Work out the finished part from the listing and answer in its coordinate system (mm). Face numbers are marked on the shaded views. A direction names the side the tool comes from. Round coordinates to 2 decimals unless told otherwise and drop trailing zeros. Loops run counter-clockwise (first coordinate to the right, second up) from the corner with the lowest first, then second, coordinate; pieces in that order, holes last. Notation, with made-up numbers: (56.25, 19.25) -> (64.25, 19.25) arc R19 ccw to (64.25, 54.25) -> close; hole circle Ø4 at (-29, 4). An arc over 180 degrees is marked (long way). Use one line per item in the form item = value.
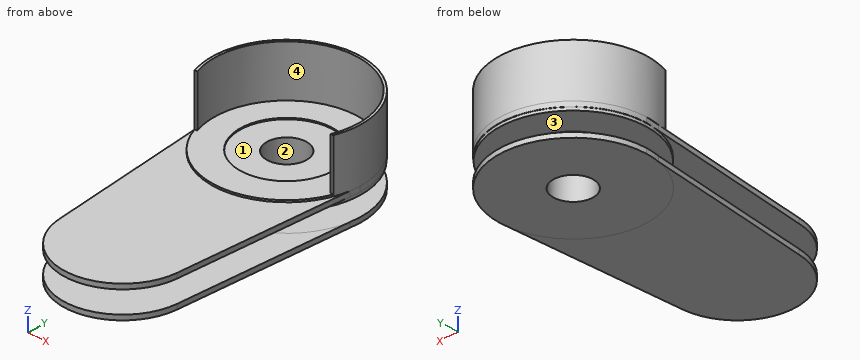
```python
from build123d import *
from build123d.topology import SkipClean

# Parameters (mm, degrees)
SKETCH2_R               = 120
BOSS_EXTRUDE2_DEPTH     = 85
CUT_EXTRUDE1_START      = -82
CUT_EXTRUDE1_DEPTH      = 82
CUT_EXTRUDE5_DEPTH      = 2
CUT_EXTRUDE5_DEPTH_BACK = 2
SKETCH8_R               = 75
SKETCH9_R               = 32
CUT_EXTRUDE6_DEPTH      = 5
BOSS_EXTRUDE4_START     = 8
SKETCH12_R              = 32
BOSS_EXTRUDE4_DEPTH     = 8
SKETCH13_R              = 119.470235088
BOSS_EXTRUDE5_DEPTH     = 5
SKETCH15_R              = 70
BOSS_EXTRUDE6_DEPTH     = 30
BOSS_EXTRUDE7_START     = 8
SKETCH16_R              = 120
BOSS_EXTRUDE7_DEPTH     = 8
CUT_EXTRUDE7_START      = -210
SKETCH19_R              = 32
CUT_EXTRUDE7_DEPTH      = 210
BOSS_EXTRUDE8_DEPTH     = 8


with BuildPart() as part:
    # Sketch2 → Boss-Extrude2 (new body)
    with BuildSketch(Plane.XY):
        Circle(SKETCH2_R)
    extrude(amount=BOSS_EXTRUDE2_DEPTH)

    # Sketch3 → Cut-Extrude1 (cut)
    with BuildSketch(Plane.XY.offset(85).offset(CUT_EXTRUDE1_START)):
        with BuildLine():
            Line((-108.885260711, -40), (-113.13708499, -40))
            ThreePointArc((-113.13708499, -40), (0, -120), (113.13708499, -40))
            Line((113.13708499, -40), (108.885260711, -40))
            ThreePointArc((108.885260711, -40), (0, 116), (-108.885260711, -40))
        make_face()
    extrude(amount=CUT_EXTRUDE1_DEPTH, mode=Mode.SUBTRACT)

    # Sketch8 → Cut-Extrude5 (cut, two sides: drawn at the far end of the back side and taken through both)
    with BuildSketch(Plane.XY.offset(3).offset(-CUT_EXTRUDE5_DEPTH_BACK)):
        Circle(SKETCH8_R)
    extrude(amount=CUT_EXTRUDE5_DEPTH + CUT_EXTRUDE5_DEPTH_BACK, mode=Mode.SUBTRACT)

    # Sketch9 → Cut-Extrude6 (cut)
    with BuildSketch(Plane.XY.offset(1)):
        Circle(SKETCH9_R)
    extrude(amount=-CUT_EXTRUDE6_DEPTH, mode=Mode.SUBTRACT)

    # Sketch12 → Boss-Extrude4 (add)
    # profile 1 of 2: a face of its own
    with SkipClean():  # the faces are left unmerged after this step: merging them gives an invalid solid
        with BuildSketch(Plane(origin=(0, 0, 0), x_dir=(-1, 0, 0), z_dir=(0, 0, -1)).offset(BOSS_EXTRUDE4_START)):
            with BuildLine():
                ThreePointArc((120, 0), (0, 120), (-120, 0))
                Line((-120, 0), (-118.831087629, -16.70845932))
                ThreePointArc((-118.831087629, -16.70845932), (-3.111785776, -119.959646504), (117.805011812, -22.84686394))
                Line((117.805011812, -22.84686394), (120, 0))
            make_face()
            with Locations(Location((0, 0, 0), (0, 0, 180))):
                Circle(SKETCH12_R, mode=Mode.SUBTRACT)
        # profile 2 of 2: a face of its own
        with BuildSketch(Plane(origin=(0, 0, 0), x_dir=(-1, 0, 0), z_dir=(0, 0, -1)).offset(BOSS_EXTRUDE4_START)):
            with BuildLine():
                ThreePointArc((117.805011812, -22.84686394), (-3.111785776, -119.959646504), (-118.831087629, -16.70845932))
                Line((-118.831087629, -16.70845932), (-99.063378042, -299.268538041))
                ThreePointArc((-99.063378042, -299.268538041), (-3.575656086, -388.008129656), (91.309922092, -298.624981255))
                Line((91.309922092, -298.624981255), (117.805011812, -22.84686394))
            make_face()
        extrude(amount=-BOSS_EXTRUDE4_DEPTH)

    # Sketch13 → Boss-Extrude5 (add)
    with SkipClean():  # the faces are left unmerged after this step: merging them gives an invalid solid
        with BuildSketch(Plane(origin=(0, 0, -8), x_dir=(-1, 0, 0), z_dir=(0, 0, -1))):
            with Locations(Location((0, 0, 0), (0, 0, 353.457468333))):
                Circle(SKETCH13_R)
        extrude(amount=BOSS_EXTRUDE5_DEPTH)

    # Sketch15 → Boss-Extrude6 (add)
    with SkipClean():  # the faces are left unmerged after this step: merging them gives an invalid solid
        with BuildSketch(Plane(origin=(0, 0, -13), x_dir=(-1, 0, 0), z_dir=(0, 0, -1))):
            Circle(SKETCH15_R)
        extrude(amount=BOSS_EXTRUDE6_DEPTH)

    # Sketch16 → Boss-Extrude7 (add)
    with BuildSketch(Plane(origin=(0, 0, -43), x_dir=(-1, 0, 0), z_dir=(0, 0, -1)).offset(BOSS_EXTRUDE7_START)):
        Circle(SKETCH16_R)
    extrude(amount=-BOSS_EXTRUDE7_DEPTH)

    # Sketch19 → Cut-Extrude7 (cut)
    with BuildSketch(Plane(origin=(0, 0, -51), x_dir=(-1, 0, 0), z_dir=(0, 0, -1)).offset(CUT_EXTRUDE7_START)):
        with Locations(Location((0, 0, 0), (0, 0, 180))):
            Circle(SKETCH19_R)
    extrude(amount=CUT_EXTRUDE7_DEPTH, mode=Mode.SUBTRACT)

    # Sketch20 → Boss-Extrude8 (add)
    with SkipClean():  # the faces are left unmerged after this step: merging them gives an invalid solid
        with BuildSketch(Plane(origin=(0, 0, -51), x_dir=(-1, 0, 0), z_dir=(0, 0, -1))):
            with BuildLine():
                ThreePointArc((117.805011812, -22.84686394), (-3.111785776, -119.959646504), (-118.831087629, -16.70845932))
                Line((-118.831087629, -16.70845932), (-99.063378042, -299.268538041))
                ThreePointArc((-99.063378042, -299.268538041), (-3.575656086, -388.008129656), (91.309922092, -298.624981255))
                Line((91.309922092, -298.624981255), (117.805011812, -22.84686394))
            make_face()
        extrude(amount=-BOSS_EXTRUDE8_DEPTH)


solid = part.part
```
(1) For the marked faces 1 and 2, determine the directions among +Z, -Z, +X, -X, +Y, -Y from which every point of the face is accessible in a straight line to the end or side of a thin tool.
Completed:
face_1 = +Z
face_2 = +Z, -Z
(2) Find section B-B, the plane x = 0. Write down the section's boundary in (y, z).
Completed:
outline = (-387.93, -51) -> (-32, -51) -> (-32, 1) -> (-75, 1) -> (-75, 3) -> (-120, 3) -> (-120, 0) -> (-387.93, 0) -> (-387.93, -8) -> (-119.47, -8) -> (-119.47, -13) -> (-70, -13) -> (-70, -43) -> (-387.93, -43) -> close; (32, -51) -> (120, -51) -> (120, -43) -> (70, -43) -> (70, -13) -> (119.47, -13) -> (119.47, -8) -> (120, -8) -> (120, 85) -> (116, 85) -> (116, 3) -> (75, 3) -> (75, 1) -> (32, 1) -> close
(3) For a pull along Y with two mould halves and no side action, classify the marked faces 3 and 4 as +Y half, -Y half, draft (parallel to the pull), parting line (faces both ways), or undercut.
Completed:
face_3 = draft
face_4 = undercut
(4) Consider L1, parallel to Y at x = 0, z = -18; L2, parallel to Z at x = -77, y = -174.5; L3, parallel to Z at x = -14.5, y = -71. Determine where each line is inside the solid, lowest interval first.
Completed:
L1 = -70 to -32, 32 to 70
L2 = -51 to -43, -8 to 0
L3 = -51 to -43, -13 to 1
(5) Find section A-A, the plane y = -287.5. Write down the section's boundary in (x, z), then the cut area to 3 significant figures.
Completed:
outline = (-92.38, -51) -> (99.89, -51) -> (99.89, -43) -> (-92.38, -43) -> close; (-92.38, -8) -> (99.89, -8) -> (99.89, 0) -> (-92.38, 0) -> close
area = 3,080 mm2
(6) Given P1, Ø8, axis at x = 81, y = -137.5, coming from the +Z side; P2, Ø1, axis at y = 43.5, z = 10, coming from the -X side; P3, Ø5, axis at x = -67, z = 6.5, coming from the +Y side, each flat-ended and moving along its own axis, determine where each tip first touches the part or whether it passes through.
Completed:
P1 = 0
P2 = -112.03
P3 = 101.19
(7) Find section C-C, the plane x = -54.5. Write down the section's boundary in (y, z).
Completed:
outline = (-368.05, -51) -> (106.91, -51) -> (106.91, -43) -> (43.93, -43) -> (43.93, -13) -> (106.32, -13) -> (106.32, -8) -> (106.91, -8) -> (106.91, 85) -> (102.4, 85) -> (102.4, 3) -> (51.52, 3) -> (51.52, 1) -> (-51.52, 1) -> (-51.52, 3) -> (-106.91, 3) -> (-106.91, 0) -> (-368.05, 0) -> (-368.05, -8) -> (-106.32, -8) -> (-106.32, -13) -> (-43.93, -13) -> (-43.93, -43) -> (-368.05, -43) -> close
(8) Find section D-D, the plane y = -58. Write down the section's boundary in (x, z).
Completed:
outline = (-114.43, -51) -> (115.94, -51) -> (115.94, -43) -> (39.19, -43) -> (39.19, -13) -> (104.45, -13) -> (104.45, -8) -> (115.94, -8) -> (115.94, 0) -> (105.05, 0) -> (105.05, 3) -> (47.55, 3) -> (47.55, 1) -> (-47.55, 1) -> (-47.55, 3) -> (-105.05, 3) -> (-105.05, 0) -> (-114.43, 0) -> (-114.43, -8) -> (-104.45, -8) -> (-104.45, -13) -> (-39.19, -13) -> (-39.19, -43) -> (-114.43, -43) -> close
